Source: CAD feature listing. Evaluate the final solid. Frame: model axes, mm. Face numbers are marked on the shaded views. Give positions to 0.01 mm unless a question says otherwise; leave off trailing zeros. Loops run counter-clockwise (first coordinate to the right, second up) from the corner with the lowest first, then second, coordinate; pieces in that order, holes last. Notation, with made-up numbers: (37.5, 80) -> (75.5, 80) arc R21 ccw to (75.5, 88) -> close; hole circle Ø6 at (88, 47.25). An arc over 180 degrees is marked (long way). Return JSON: item names as keys, results as strings. Group by question number.
(1) Cut plane C-C on x = 160. Return loops of the section in (y, z).
(2) Pin query (flat end, axial travel): pin 1 (1 mm diameter, centred on x = 48.5, z = -88.5, fed in from -Y); pin 2 (8 mm diameter, centred on x = 43.5, z = -185, fed in from -Y); pin 3 (6 mm diameter, centred on x = 59.5, y = 229.5, fed in from -Z). Return the tip coordinate at first contact, or that it passes through.
(3) Draft query along Z for the marked faces 1 and 2. Return one class per face: released by +Z, released by -Z, zero draft, split by the parting line, or undercut.
(4) Cut plane A-A on y = 0. Return loops of the section in (x, z).
(5) Ray query, line 1 (Y direction, x = -4.5, z = -393.5); line 2 (Y direction, x = -41, z = -354); line 3 (Z direction, x = 70.5, y = 241). Return the intervals inside material, ascending. Write a range as from..to.
(6) Cut plane B-B on x = 57. Return loops of the section in (y, z), then the cut area to 3 significant figures.
```python
from build123d import *


# Not quite as in the source:
# - the program builds the solid bodies; features that only make, move or delete a surface that nothing else refers to are left out


with BuildPart() as f4:
    # F0 (on Front) → F4 (revolve)
    with BuildSketch(Plane.XZ):
        with BuildLine():
            ThreePointArc((-192.4457153976, -49.2647496334), (-177.5667398819, -85.1857741176), (-141.6457153976, -100.0647496334))
            Line((-141.6457153976, -100.0647496334), (137.7542846024, -100.0647496334))
            ThreePointArc((137.7542846024, -100.0647496334), (173.6753090867, -85.1857741176), (188.5542846024, -49.2647496334))
            Line((188.5542846024, -49.2647496334), (188.5542846024, 1.5352503666))
            ThreePointArc((188.5542846024, 1.5352503666), (173.6753090867, 37.4562748509), (137.7542846024, 52.3352503666))
            Line((137.7542846024, 52.3352503666), (-141.6457153976, 52.3352503666))
            ThreePointArc((-141.6457153976, 52.3352503666), (-177.5667398819, 37.4562748509), (-192.4457153976, 1.5352503666))
            Line((-192.4457153976, 1.5352503666), (-192.4457153976, -49.2647496334))
        make_face()
    revolve(axis=Axis((-11.0372006893, 0, -386.9243860245), (-1, 0, 0)))


solid = f4.part
```
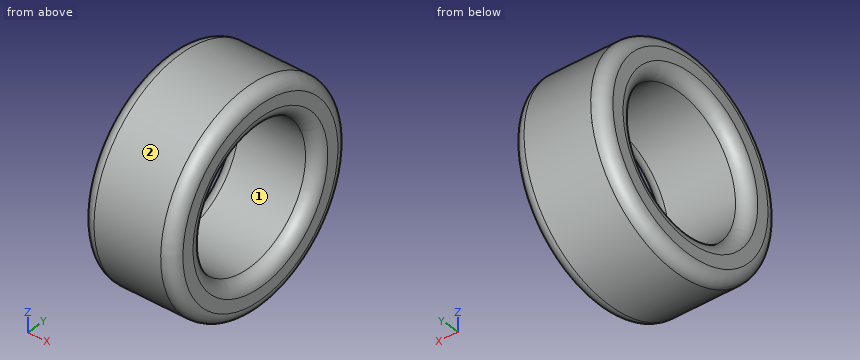
Answers:
{
 "1": {"outline": "circle Ø868.26 at (0, -386.92); hole circle Ø583.98 at (0, -386.92)"},
 "2": {"pin 1": "y = -322.78", "pin 2": "y = -392.14", "pin 3": "z = -763.28"},
 "3": {"face 1": "undercut", "face 2": "split by the parting line"},
 "4": {"outline": "(-192.45, -775.38) arc R50.8 ccw to (-141.65, -826.18) -> (137.75, -826.18) arc R50.8 ccw to (188.55, -775.38) -> (188.55, -724.58) arc R50.8 ccw to (137.75, -673.78) -> (-141.65, -673.78) arc R50.8 ccw to (-192.45, -724.58) -> close; (-192.45, -49.26) arc R50.8 ccw to (-141.65, -100.06) -> (137.75, -100.06) arc R50.8 ccw to (188.55, -49.26) -> (188.55, 1.54) arc R50.8 ccw to (137.75, 52.34) -> (-141.65, 52.34) arc R50.8 ccw to (-192.45, 1.54) -> close"},
 "5": {"line 1": "-439.21..-286.78, 286.78..439.21", "line 2": "-438.02..-284.96, 284.96..438.02", "line 3": "-754.17..-542.51, -231.34..-19.68"},
 "6": {"outline": "circle Ø878.52 at (0, -386.92); hole circle Ø573.72 at (0, -386.92)", "area": "348,000 mm²"}
}
